from build123d import *

# Parameters (mm, degrees)
ESQUISSE1_R        = 1.25
BOSS_EXTRU_1_DEPTH = 11.5
BOSS_EXTRU_2_DEPTH = 2


with BuildPart() as part:
    # Esquisse1 → Boss.-Extru.1 (new body)
    with BuildSketch(Plane.XY):
        Circle(ESQUISSE1_R)
    extrude(amount=BOSS_EXTRU_1_DEPTH)

    # Esquisse2 → Boss.-Extru.2 (add)
    with BuildSketch(Plane(origin=(0, 0, 0), x_dir=(-1, 0, 0), z_dir=(0, 0, -1))):
        Polygon((0, 2.5), (-2.165063509, 1.25), (-2.165063509, -1.25), (0, -2.5), (2.165063509, -1.25), (2.165063509, 1.25), align=None)
    extrude(amount=BOSS_EXTRU_2_DEPTH)


solid = part.part
Geometry: final body of the model. Coordinates: model frame, mm. A direction names the side the tool comes from. Round coordinates to 2 decimals unless told otherwise and drop trailing zeros. Loops run counter-clockwise (first coordinate to the right, second up) from the corner with the lowest first, then second, coordinate; pieces in that order, holes last. Notation, with made-up numbers: (-18, 71) -> (-8, 71) arc R32 cw to (-8, 103) -> close; hole circle Ø11 at (-9.75, -3.75). An arc over 180 degrees is marked (long way). One line per question, with ' | ' between items. Start each with the question number.
1. Set-up query: faces 1 (the face through (-1.098, 1.866, -0.986)), 2 (the face through (1, -1, 0)). Return all of +Z, -Z, +X, -X, +Y, -Y with unobstructed straight access to the full face (end or side cutting, diameter ignored); none if empty.
2. Section A-A on y = 0. Output: boundary loops of the cut face in (x, z).
3. Section C-C on z = 9.25. Output: boundary loops of the cut face in (x, y).
4. Line query: line 1 along Z through (x, y) = (1.7, -0.6); line 2 along Y through (x, z) = (0.05, 5.25); line 3 along Y through (x, z) = (0.85, 3.75). Output: solid intervals per line, ascending. Write a range as [from, to].
5. Section D-D on x = 1.6. Output: boundary loops of the cut face in (y, z), and give its area (3 significant figures).
6. Section B-B on x = -0.95. Output: boundary loops of the cut face in (y, z).
7. Contact query for a flat-ended pin moving along its axis: pin 1 (1 mm diameter, centred on y = 0.5, z = 5, fed in from +X). Output: stop coordinate, or through.
Returned:
1) face 1: +Z, -Z, -X, +Y | face 2: +Z
2) outline: (-2.17, -2) -> (2.17, -2) -> (2.17, 0) -> (1.25, 0) -> (1.25, 11.5) -> (-1.25, 11.5) -> (-1.25, 0) -> (-2.17, 0) -> close
3) outline: circle Ø2.5 at (0, 0)
4) line 1: z = [-2, 0] | line 2: y = [-1.25, 1.25] | line 3: y = [-0.92, 0.92]
5) outline: (-1.58, -2) -> (1.58, -2) -> (1.58, 0) -> (-1.58, 0) -> close | area: 6.30 mm2
6) outline: (-1.95, -2) -> (1.95, -2) -> (1.95, 0) -> (0.81, 0) -> (0.81, 11.5) -> (-0.81, 11.5) -> (-0.81, 0) -> (-1.95, 0) -> close
7) pin 1: stops at x = 1.25
